from build123d import *

# Parameters (mm, degrees)
F1_DEPTH = 90.17
F0_W     = 25.4
F0_H     = 19.05
F2_DEPTH = 25.4
F3_DEPTH = 7.9375


with BuildPart() as f1:
    # F0 (on Front) → F1 (new body, symmetric)
    with BuildSketch(Plane.XZ):
        Polygon((41.275, -9.525), (41.275, 9.525), (22.225, 9.525), (-41.275, 9.525), (-41.275, -9.525), align=None)
    extrude(amount=F1_DEPTH, both=True)

    # F0 (on Front) → F2 (join, symmetric)
    with BuildSketch(Plane.XZ):
        with BuildLine():
            Line((22.225, 9.525), (41.275, 9.525))
            Line((41.275, 9.525), (41.275, 27.0002))
            ThreePointArc((41.275, 27.0002), (45.9246798487, 38.2255201513), (57.15, 42.8752))
            Line((57.15, 42.8752), (60.325, 42.8752))
            Line((60.325, 42.8752), (60.325, 61.9252))
            Line((60.325, 61.9252), (57.15, 61.9252))
            ThreePointArc((57.15, 61.9252), (32.4542956671, 51.6959043329), (22.225, 27.0002))
            Line((22.225, 27.0002), (22.225, 9.525))
        make_face()
        with Locations((73.025, 52.4002)):
            Rectangle(F0_W, F0_H)
    extrude(amount=F2_DEPTH, both=True)

    # F0 (on Front) → F3 (join, symmetric)
    with BuildSketch(Plane.XZ):
        with BuildLine():
            Line((-41.275, 9.525), (22.225, 9.525))
            Line((22.225, 9.525), (22.225, 27.0002))
            ThreePointArc((22.225, 27.0002), (32.4542956671, 51.6959043329), (57.15, 61.9252))
            add(Edge.make_bspline(
                [(-41.275, 9.525), (-35.8186467643, 28.3691705971), (4.2723575607, 65.0347471237), (57.15, 61.9252)],
                knots=[0, 0, 0, 0, 111.5045361635, 111.5045361635, 111.5045361635, 111.5045361635], degree=3))
        make_face()
    extrude(amount=F3_DEPTH, both=True)


solid = f1.part
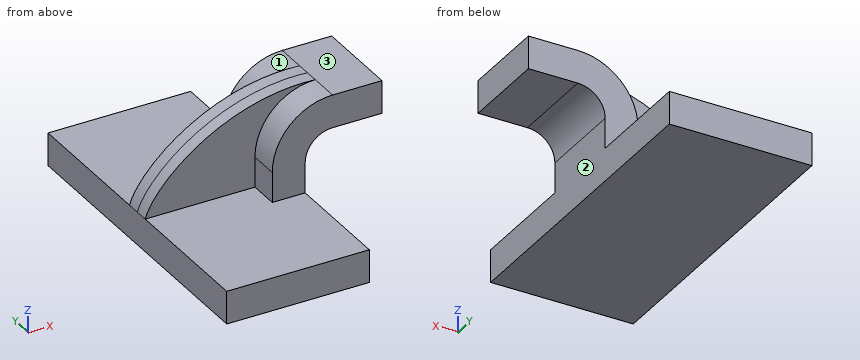
Source: CAD feature listing. Evaluate the final solid. Frame: model axes, mm. Face numbers are marked on the shaded views. A direction names the side the tool comes from. Coordinates: 2 decimals unless noted, no trailing zeros. Loops run counter-clockwise (first coordinate to the right, second up) from the corner with the lowest first, then second, coordinate; pieces in that order, holes last. Notation, with made-up numbers: (50.25, 5) -> (88.25, 5) arc R31 cw to (88.25, 40) -> close; hole circle Ø7 at (-10.75, -15.5). An arc over 180 degrees is marked (long way). Answer in a Markdown table with one row per item. Add a question column.
Q1. Reachability of the marked faces 1, 2 and 3 from +Z, -Z, +X, -X, +Y, -Y: full face, straight path, thin tool, end or side. Return the list, or none.
Q2. Section C-C on x = 78. Return the cut outline in (y, z), and give its area (3 significant figures).
Q3. Contact query for flat-ended pins moving along their axis: pin 1 Ø2 at (x, z) = (31.5, 54) entering from -Y; pin 2 Ø5 at (y, z) = (19.5, 14.5) entering from -X (3 decimals); pin 3 Ø1.5 at (y, z) = (70.5, 6.5) entering from +X (3 decimals). Output: stop coordinate, or through.
Q4. Section A-A on y = -10.5. Return the cut outline in (x, z) (3 decimals), and give its area (3 significant figures).
Q5. Ray query, line 1 along Y through (x, z) = (74, 58); line 2 along Z through (x, y) = (-30.5, 50.5) (3 decimals); line 3 along Y through (x, z) = (19.5, 45). Return the intervals inside material, ascending.
Computed values:
| question | item | result |
|---|---|---|
| 1 | face 1 | +Z, -X, +Y |
| 1 | face 2 | -Z, +X, +Y, -Y |
| 1 | face 3 | +Z, +X, +Y, -Y |
| 2 | outline | (-25.4, 42.88) -> (25.4, 42.88) -> (25.4, 61.93) -> (-25.4, 61.93) -> close |
| 2 | area | 968 mm^2 |
| 3 | pin 1 | stops at y = -7.94 |
| 3 | pin 2 | stops at x = 22.225 |
| 3 | pin 3 | stops at x = 41.275 |
| 4 | outline | (-41.275, -9.525) -> (41.275, -9.525) -> (41.275, 27) arc R15.875 cw to (57.15, 42.875) -> (85.725, 42.875) -> (85.725, 61.925) -> (57.15, 61.925) arc R34.925 ccw to (22.225, 27) -> (22.225, 9.525) -> (-41.275, 9.525) -> close |
| 4 | area | 3,210 mm^2 |
| 5 | line 1 | y = -25.4 to 25.4 |
| 5 | line 2 | z = -9.525 to 9.525 |
| 5 | line 3 | y = -7.94 to 7.94 |
